The listing builds one solid part. Answer for the finished solid, in the listing's coordinates (mm). A direction names the side the tool comes from. Coordinates: 2 decimals unless noted, no trailing zeros. Order: outer loops, then holes, each group sorted by start corner. A loop starts at its lowest first (then second) coordinate and runs counter-clockwise, first axis right, second up. Notation, with made-up numbers: (-20, -4.75) - (5, -4.75) arc R28 ccw to (5, 25.25) - close; hole circle Ø8 at (41.25, 48). An arc over 180 degrees is marked (long way). Use a Markdown table: item, result. Add a question column.
Item 1: The part is cut by section B-B, the plane y = 8. Give the vertices of the cut face in (x, z).
Item 2: Find the intervals of material crossed by line 1 along Z through (x, y) = (-11.5, -0.5); line 2 along X through (y, z) = (3.5, 1.7); line 3 along X through (y, z) = (6.75, 3.05), in increasing order.
Item 3: The part is cut by section C-C, the plane y = -6.75. Give the vertices of the cut face in (x, z), then the cut area to 3 significant figures.
Item 4: The mould has two halves that part along Z. Classify faces 4 (the flat face through (0, 10, 1)), 5 (the flat face through (-10, 2, 1.5)), 6 (the flat face through (0, -5, 2)), 7 (the flat face through (0, 0, 0)): released by +Z, released by -Z, zero draft, split by the parting line, or undercut.
Item 5: The part is cut by section A-A, the plane x = 3.5. Give the vertices of the cut face in (y, z).
Item 6: Flat-ended cylindrical pins translate along their axes: P1, Ø11, axis at x = -1.5, y = -2.5, coming from the -Z side; P2, Ø11, axis at x = 5.5, y = -6.5, coming from the +Z side; P3, Ø0.5, axis at x = -10, z = 1.5, coming from the +Y side. Find the tip coordinate at first contact, or state that the pin passes through.
Item 7: For faces 1 (the flat face through (0, -5, 1)), 2 (the flat face through (-0.3, -10, 2.5)), 3 (the flat face through (10, 2, 1.5)), determine the directions among +Z, -Z, +X, -X, +Y, -Y from which every point of the face is accessible in a straight line to the end or side of a thin tool.
Item 8: The part is cut by section D-D, the plane y = 0.5. Give the vertices of the cut face in (x, z), then the cut area to 3 significant figures.
from build123d import *

# Parameters (mm, degrees)
F0_W     = 40
F0_H     = 20
F1_DEPTH = 3
F2_W     = 40
F2_H     = 1
F3_DEPTH = 10
F5_DEPTH = 10
F6_DEPTH = 8


with BuildPart() as f1:
    # F0 (on Top) → F1 (new body)
    with BuildSketch(Plane.XY):
        Rectangle(F0_W, F0_H)
    extrude(amount=F1_DEPTH)

    # F2 (on face) → F3 (cut)
    with BuildSketch(Plane.XZ.offset(10)):
        with Locations((0, 1.5)):
            Rectangle(F2_W, F2_H)
    extrude(amount=-F3_DEPTH, mode=Mode.SUBTRACT)

    # F4 (on face) → F5 (join)
    with BuildSketch(Plane(origin=(0, 10, 0), x_dir=(-1, 0, 0), z_dir=(0, 1, 0))):
        with BuildLine():
            ThreePointArc((10, 3.5), (9.2928932188, 3.3708286934), (8.6771243445, 3))
            Line((8.6771243445, 3), (10, 3))
            Line((10, 3), (10, 3.5))
        make_face()
        with BuildLine():
            Line((-10, 3), (-8.6771243445, 3))
            ThreePointArc((-8.6771243445, 3), (-9.2928932188, 3.3708286934), (-10, 3.5))
            Line((-10, 3.5), (-10, 3))
        make_face()
        with BuildLine():
            ThreePointArc((11.3228756555, 3), (10.7071067812, 3.3708286934), (10, 3.5))
            Line((10, 3.5), (10, 3))
            Line((10, 3), (11.3228756555, 3))
        make_face()
        with BuildLine():
            Line((-10, 3), (-10, 3.5))
            ThreePointArc((-10, 3.5), (-10.7071067812, 3.3708286934), (-11.3228756555, 3))
            Line((-11.3228756555, 3), (-10, 3))
        make_face()
        with BuildLine():
            ThreePointArc((-10, -0.5), (-9.2928932188, -0.3708286934), (-8.6771243445, 0))
            Line((-8.6771243445, 0), (-10, 0))
            Line((-10, 0), (-10, -0.5))
        make_face()
        with BuildLine():
            Line((10, 0), (8.6771243445, 0))
            ThreePointArc((8.6771243445, 0), (9.2928932188, -0.3708286934), (10, -0.5))
            Line((10, -0.5), (10, 0))
        make_face()
        with BuildLine():
            ThreePointArc((-11.3228756555, 0), (-10.7071067812, -0.3708286934), (-10, -0.5))
            Line((-10, -0.5), (-10, 0))
            Line((-10, 0), (-11.3228756555, 0))
        make_face()
        with BuildLine():
            Line((10, 0), (10, -0.5))
            ThreePointArc((10, -0.5), (10.7071067812, -0.3708286934), (11.3228756555, 0))
            Line((11.3228756555, 0), (10, 0))
        make_face()
    extrude(amount=-F5_DEPTH)

    # F4 (on face) → F6 (cut)
    with BuildSketch(Plane(origin=(0, 10, 0), x_dir=(-1, 0, 0), z_dir=(0, 1, 0))):
        with BuildLine():
            ThreePointArc((-10, 2), (-10.5, 1.5), (-10, 1))
            Line((-10, 1), (-10, 2))
        make_face()
        with BuildLine():
            Line((-10, 2), (-10, 1))
            ThreePointArc((-10, 1), (-9.6464466094, 1.1464466094), (-9.5, 1.5))
            ThreePointArc((-9.5, 1.5), (-9.6464466094, 1.8535533906), (-10, 2))
        make_face()
        with BuildLine():
            Line((10, 2), (10, 1))
            ThreePointArc((10, 1), (10.3535533906, 1.1464466094), (10.5, 1.5))
            ThreePointArc((10.5, 1.5), (10.3535533906, 1.8535533906), (10, 2))
        make_face()
        with BuildLine():
            ThreePointArc((10, 2), (9.5, 1.5), (10, 1))
            Line((10, 1), (10, 2))
        make_face()
    extrude(amount=-F6_DEPTH, mode=Mode.SUBTRACT)


solid = f1.part
Solution:
| question | item | result |
|---|---|---|
| 1 | outline | (-20, 0) - (-11.32, 0) arc R2 ccw to (-8.68, 0) - (8.68, 0) arc R2 ccw to (11.32, 0) - (20, 0) - (20, 3) - (11.32, 3) arc R2 ccw to (8.68, 3) - (-8.68, 3) arc R2 ccw to (-11.32, 3) - (-20, 3) - close; hole circle Ø1 at (-10, 1.5); hole circle Ø1 at (10, 1.5) |
| 2 | line 1 | z = 0 to 1, 2 to 3 |
| 2 | line 2 | x = -20 to -10.46, -9.54 to 9.54, 10.46 to 20 |
| 2 | line 3 | x = -11.26 to -8.74, 8.74 to 11.26 |
| 3 | outline | (-20, 0) - (20, 0) - (20, 1) - (-20, 1) - close; (-20, 2) - (20, 2) - (20, 3) - (-20, 3) - close |
| 3 | area | 80.0 mm2 |
| 4 | face 4 | zero draft |
| 4 | face 5 | undercut |
| 4 | face 6 | undercut |
| 4 | face 7 | released by -Z |
| 5 | outline | (-10, 0) - (10, 0) - (10, 3) - (-10, 3) - (-10, 2) - (0, 2) - (0, 1) - (-10, 1) - close |
| 6 | P1 | stops at z = 0 |
| 6 | P2 | stops at z = 3 |
| 6 | P3 | stops at y = 2 |
| 7 | face 1 | +X, -X, -Y |
| 7 | face 2 | +Z, -Z, +X, -X, -Y |
| 7 | face 3 | +Y |
| 8 | outline | (-20, 0) - (-11.32, 0) arc R2 ccw to (-8.68, 0) - (8.68, 0) arc R2 ccw to (11.32, 0) - (20, 0) - (20, 3) - (11.32, 3) arc R2 ccw to (8.68, 3) - (-8.68, 3) arc R2 ccw to (-11.32, 3) - (-20, 3) - close |
| 8 | area | 124 mm2 |
